Verification items for this drawing (mm, ordinates from the low corner). A direction names the side the tool comes from. Round coordinates to 2 decimals unless told otherwise and drop trailing zeros. Loops run counter-clockwise (first coordinate to the right, second up) from the corner with the lowest first, then second, coordinate; pieces in that order, holes last. Notation, with made-up numbers: (2, -1.5) - (37, -1.5) arc R6 ccw to (37, 5.5) - close; hole circle Ø10 at (83.5, 59.5). An arc over 180 degrees is marked (long way). Answer in a Markdown table with one row per item. Add a question column.
(1) Gauge pin test, flat ends, axial feed: pin 1 (1 mm diameter, centred on y = 1, z = 3, fed in from -X) (1 decimal); pin 2 (1.5 mm diameter, centred on x = 3, y = 4.5, fed in from -Z); pin 3 (1.5 mm diameter, centred on y = 3.5, z = 2, fed in from -X). Record the tip position at first contact, or that the pin passes through.
(2) Access from +Z, -Z, +X, -X, +Y, -Y to the whole of each face (thin tool, end or side, straight path). Record for the marked faces 1 and 2.
(3) Thickness scan on line 1 along X through (y, z) = (5, 7.75) (1 decimal); line 2 along Y through (x, z) = (8.5, 1) (1 decimal); line 3 along Z through (x, y) = (7.25, 4.4). Record the ranges inside material, lowest first.
(4) Cross-section at C-C on y = 1.7. Enter the section's corners in (x, z) (1 decimal).
(5) Mould release check, pull along Z, two halves, no side actions. Record for the marked faces 3, 4 and 5: +Z half, -Z half, draft (parallel to the pull), parting line (faces both ways), or undercut.
(6) Cross-section at A-A on z = 8.5. Enter the section's corners in (x, y) (1 decimal).
(7) Cross-section at B-B on x = 2.75. Enter the section's corners in (y, z) (1 decimal).
(8) Cross-section at D-D on y = 2.8. Enter the section's corners in (x, z) (1 decimal).
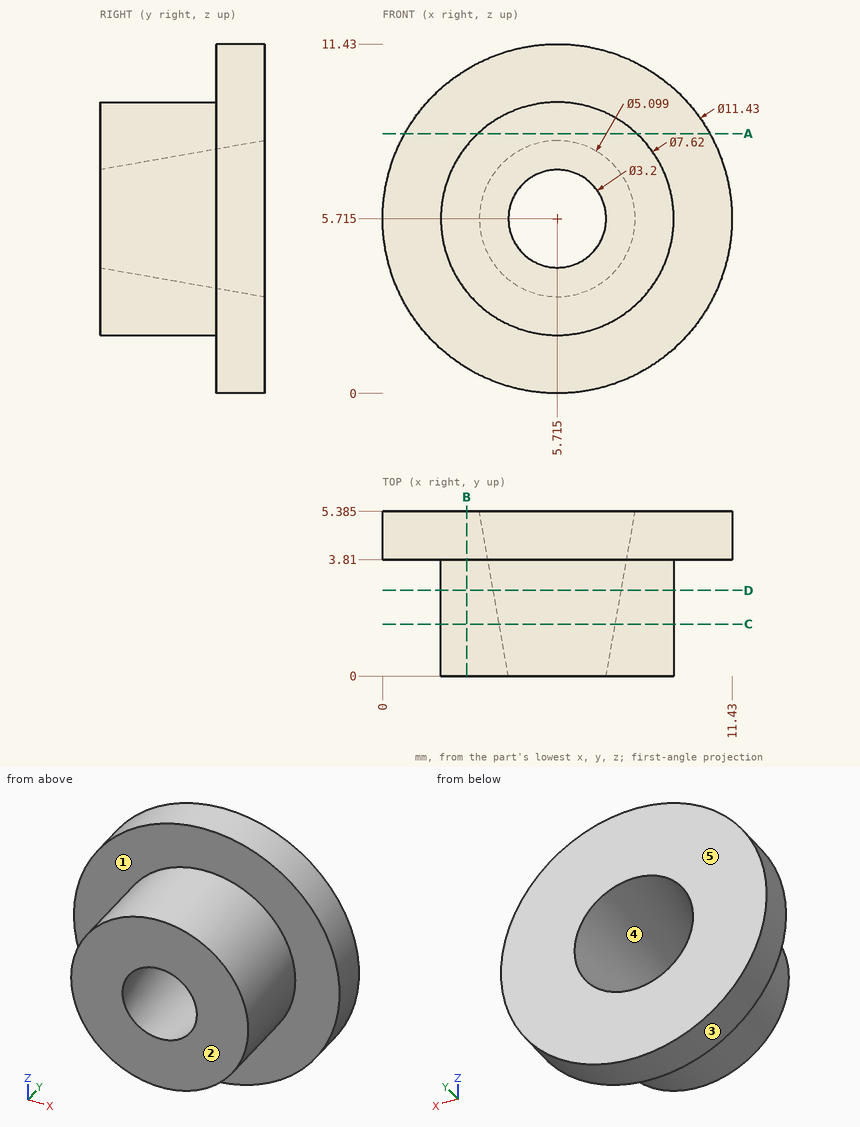
Answers:
| question | item | result |
|---|---|---|
| 1 | pin 1 | stops at x = 2.6 |
| 1 | pin 2 | stops at z = 0.35 |
| 1 | pin 3 | stops at x = 0.87 |
| 2 | face 1 | -Y |
| 2 | face 2 | +Z, -Z, +X, -X, -Y |
| 3 | line 1 | x = 0.4 to 4.3, 7.1 to 11.1 |
| 3 | line 2 | y = 3.8 to 5.4 |
| 3 | line 3 | z = 0.21 to 3.9, 7.53 to 11.22 |
| 4 | outline | circle Ø7.6 at (5.7, 5.7); hole circle Ø3.8 at (5.7, 5.7) |
| 5 | face 3 | parting line |
| 5 | face 4 | undercut |
| 5 | face 5 | draft |
| 6 | outline | (0.7, 3.8) - (3.1, 3.8) - (3.1, 0) - (8.3, 0) - (8.3, 3.8) - (10.7, 3.8) - (10.7, 5.4) - (0.7, 5.4) - close |
| 7 | outline | (0, 3.3) - (3.8, 3.3) - (3.8, 0.8) - (5.4, 0.8) - (5.4, 10.6) - (3.8, 10.6) - (3.8, 8.1) - (0, 8.1) - close |
| 8 | outline | circle Ø7.6 at (5.7, 5.7); hole circle Ø4.2 at (5.7, 5.7) |
